Read the model definition and answer for the solid it produces. Units are mm, in the model's axes. Face numbers are marked on the shaded views. A direction names the side the tool comes from. Round coordinates to 2 decimals unless told otherwise and drop trailing zeros. Loops run counter-clockwise (first coordinate to the right, second up) from the corner with the lowest first, then second, coordinate; pieces in that order, holes last. Notation, with made-up numbers: M 72,31 L 78,31 A12 ccw 78,49 Z; hole C 17.5,-25 d9. An arc over 180 degrees is marked long. Write each question's results on one line, items separated by ' | '.
from build123d import *

# Parameters (mm, degrees)
SKETCH1_W           = 7.1
SKETCH1_H           = 11.1
SKETCH1_W_2         = 5.1
SKETCH1_H_2         = 9.1
SKETCH1_H_3         = 8
BOSS_EXTRUDE1_DEPTH = 3


with BuildPart() as part:
    # Sketch1 → Boss-Extrude1 (new body)
    # profile 1 of 2: a face of its own
    with BuildSketch(Plane(origin=(0, 0, 0), x_dir=(1, 0, 0), z_dir=(0, 1, 0))):
        with Locations((2.55, -4.55)):
            Rectangle(SKETCH1_W, SKETCH1_H)
        with Locations((2.55, -4.55)):
            Rectangle(SKETCH1_W_2, SKETCH1_H_2, mode=Mode.SUBTRACT)
    # profile 2 of 2: a face of its own
    with BuildSketch(Plane(origin=(0, 0, 0), x_dir=(1, 0, 0), z_dir=(0, 1, 0))):
        with Locations((2.55, -14.1)):
            Rectangle(SKETCH1_W, SKETCH1_H_3)
    extrude(amount=BOSS_EXTRUDE1_DEPTH)


solid = part.part
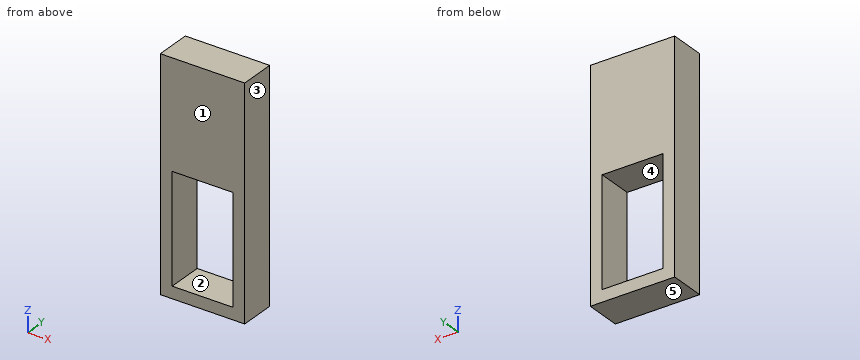
Item 1: A flat-ended cylindrical pin translates along its axis: pin 1 (3 mm diameter, centred on x = 2.5, z = 4, fed in from +Y). Find the tip coordinate at first contact, or state that the pin passes through.
Outcome:
pin 1: passes through
Item 2: For the marked faces 4 and 5, determine the directions among +Z, -Z, +X, -X, +Y, -Y from which every point of the face is accessible in a straight line to the end or side of a thin tool.
Outcome:
face 4: +Y, -Y | face 5: -Z, +X, -X, +Y, -Y
Item 3: Straight lines are drawn through the part: line 1 (X direction, y = 1.4, z = 8.5); line 2 (Z direction, x = 4.75, y = 2.55). For each, find the intervals that lie inside material, in ascending order.
Outcome:
line 1: x = -1 to 0, 5.1 to 6.1 | line 2: z = -1 to 0, 9.1 to 18.1
Item 4: The mould has two halves that part along X. Classify the marked faces 1, 2 and 3: pulls with the +X half, pulls with the -X half, needs draft (parallel to the pull), parting line crosses it, or undercut.
Outcome:
face 1: needs draft | face 2: undercut | face 3: pulls with the +X half
Item 5: The part is cut by section B-B (x = 3.5). Determine the outline of the cut face in (y, z), plus the area to 3 significant figures.
Outcome:
outline: M 0,-1 L 3,-1 L 3,0 L 0,0 Z; M 0,9.1 L 3,9.1 L 3,18.1 L 0,18.1 Z | area: 30.0 mm2
Item 6: The part is cut by section C-C (y = 2.45). Determine the outline of the cut face in (x, z).
Outcome:
outline: M -1,-1 L 6.1,-1 L 6.1,18.1 L -1,18.1 Z; hole M 0,0 L 5.1,0 L 5.1,9.1 L 0,9.1 Z
Item 7: The part is cut by section A-A (z = 7.75). Determine the outline of the cut face in (x, y), plus the area to 3 significant figures.
Outcome:
outline: M -1,0 L 0,0 L 0,3 L -1,3 Z; M 5.1,0 L 6.1,0 L 6.1,3 L 5.1,3 Z | area: 6.00 mm2
